from build123d import *

# Parameters (mm, degrees)
SKIZZE1_W                       = 13
SKIZZE1_H                       = 13
AUFSATZ_LINEAR_AUSTRAGEN1_DEPTH = 11
WANDUNG1_T                      = -1
SKIZZE2_W                       = 1
SKIZZE2_H                       = 7
SCHNITT_LINEAR_AUSTRAGEN1_DEPTH = 12


with BuildPart() as part:
    # Skizze1 → Aufsatz-Linear austragen1 (new body)
    with BuildSketch(Plane(origin=(0, 0, 0), x_dir=(0, 0, -1), z_dir=(1, 0, 0))):
        with Locations((6.5, 6.5)):
            Rectangle(SKIZZE1_W, SKIZZE1_H)
    extrude(amount=AUFSATZ_LINEAR_AUSTRAGEN1_DEPTH)

    # Wandung1
    wandung1_openings = [part.faces().sort_by_distance(p)[0] for p in [
        (5.5, 6.5, 0),
    ]]
    offset(amount=WANDUNG1_T, openings=wandung1_openings, kind=Kind.INTERSECTION)

    # Skizze2 → Schnitt-Linear austragen1 (cut)
    with BuildSketch(Plane.XY):
        with Locations((0.5, 6.5)):
            Rectangle(SKIZZE2_W, SKIZZE2_H)
    extrude(amount=-SCHNITT_LINEAR_AUSTRAGEN1_DEPTH, mode=Mode.SUBTRACT)


solid = part.part
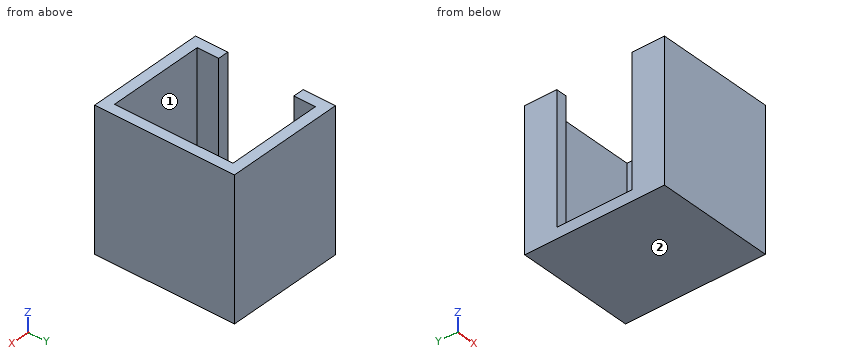
Input: part model. Units: mm. Frame: model coordinates. Face numbers are marked on the shaded views. A direction names the side the tool comes from. Round coordinates to 2 decimals unless told otherwise and drop trailing zeros. Loops run counter-clockwise (first coordinate to the right, second up) from the corner with the lowest first, then second, coordinate; pieces in that order, holes last. Notation, with made-up numbers: (15.25, 74.5) -> (38.25, 74.5) arc R10 cw to (38.25, 86.5) -> close; hole circle Ø5 at (-40, 35). An arc over 180 degrees is marked (long way). Answer as a JSON object with one key per item and string values. Group by question number.
1) Section query D-D on y = 8. Output: boundary loops of the cut face in (x, z).
2) Reachability of the marked faces 1 and 2 from +Z, -Z, +X, -X, +Y, -Y: full face, straight path, thin tool, end or side. Return the list, or none.
3) Pin query (flat end, axial travel): pin 1 (4.5 mm diameter, centred on x = 4.5, z = -3.5, fed in from -Y). Return the tip coordinate at first contact, or that it passes through.
4) Section query A-A on x = 4.25. Output: boundary loops of the cut face in (y, z), plus the area to 3 significant figures.
5) Section query C-C on z = -1.5. Output: boundary loops of the cut face in (x, y), plus the area to 3 significant figures.
6) Ray query, L1, parallel to X at y = 2.75, z = -8; L2, parallel to Y at x = 8.25, z = -6; L3, parallel to Z at x = 9.5, y = 5.75. Return the intervals inside material, ascending.
7) Section query B-B on y = 11.25. Output: boundary loops of the cut face in (x, z), plus the area to 3 significant figures.
Reply:
{
 "1": {"outline": "(0, -13) -> (11, -13) -> (11, 0) -> (10, 0) -> (10, -12) -> (0, -12) -> close"},
 "2": {"face 1": "+Z", "face 2": "-Z, +X, -X, +Y, -Y"},
 "3": {"pin 1": "stops at y = 0"},
 "4": {"outline": "(0, -13) -> (13, -13) -> (13, 0) -> (12, 0) -> (12, -12) -> (1, -12) -> (1, 0) -> (0, 0) -> close", "area": "37.0 mm2"},
 "5": {"outline": "(0, 0) -> (11, 0) -> (11, 13) -> (0, 13) -> (0, 10) -> (1, 10) -> (1, 12) -> (10, 12) -> (10, 1) -> (1, 1) -> (1, 3) -> (0, 3) -> close", "area": "37.0 mm2"},
 "6": {"L1": "x = 0 to 1, 10 to 11", "L2": "y = 0 to 1, 12 to 13", "L3": "z = -13 to -12"},
 "7": {"outline": "(0, -13) -> (11, -13) -> (11, 0) -> (10, 0) -> (10, -12) -> (1, -12) -> (1, 0) -> (0, 0) -> close", "area": "35.0 mm2"}
}
